CAD build for the part. Positions are in the model's coordinates, mm. Face numbers are marked on the shaded views. A direction names the side the tool comes from. Coordinates: 2 decimals unless noted, no trailing zeros. Answer as CSV lines item,"result". Start each with the question number.
```python
from build123d import *

# Parameters (mm, degrees)
CHAMFER1_SIZE       = 0.5
CHAMFER2_SIZE       = 0.8
SKETCH3_R           = 40.418258265
SKETCH3_R_2         = 4.375
BOSS_EXTRUDE1_DEPTH = 6.7
CHAMFER3_SIZE       = 1.5


with BuildPart() as part:
    # Sketch1 → Revolve1 (revolve)
    with BuildSketch(Plane(origin=(0, 0, 0), x_dir=(1, 0, 0), z_dir=(0, 1, 0)), mode=Mode.PRIVATE) as revolve1_sk:
        Polygon((37.9, 0), (37.9, -8.7), (48, -8.7), (48, -18.7), (51, -18.7), (51, -16.2), (50, -16.2), (50, -11.2), (51, -11.2), (51, -8.7), (52, -8.7), (52, -6.7), (39.9, -6.7), (39.9, 0), align=None)
    revolve(revolve1_sk.sketch.rotate(Axis((0, 0, -73.981367368), (0, 0, 1)), 180), axis=Axis((0, 0, -73.981367368), (0, 0, 1)))

    # Chamfer1
    chamfer1_edges = [part.edges().sort_by_distance(p)[0] for p in [
        (51, 0, 11.2),
        (50, 0, 11.2),
        (50, 0, 16.2),
        (51, 0, 16.2),
        (51, 0, 18.7),
        (39.9, 0, 0),
    ]]
    chamfer(chamfer1_edges, length=CHAMFER1_SIZE - 0.0001)  # a hair under: the kernel refuses the full size

    # Chamfer2
    chamfer2_edges = [part.edges().sort_by_distance(p)[0] for p in [
        (51, 0, 8.7),
    ]]
    chamfer(chamfer2_edges, length=CHAMFER2_SIZE)

    # Sketch3 → Boss-Extrude1 (add)
    with BuildSketch(Plane(origin=(0, 0, 6.7), x_dir=(-1, 0, 0), z_dir=(0, 0, -1))):
        with Locations(Location((0.518258265, 0, 0), (0, 0, 180))):
            Circle(SKETCH3_R)
        with Locations(Location((0.518258265, 0, 0), (0, 0, 180))):
            Circle(SKETCH3_R_2, mode=Mode.SUBTRACT)
    extrude(amount=BOSS_EXTRUDE1_DEPTH)

    # Chamfer3
    chamfer3_edges = [part.edges().sort_by_distance(p)[0] for p in [
        (-4.893258265, 0, 0),
    ]]
    chamfer(chamfer3_edges, length=CHAMFER3_SIZE)


solid = part.part
```
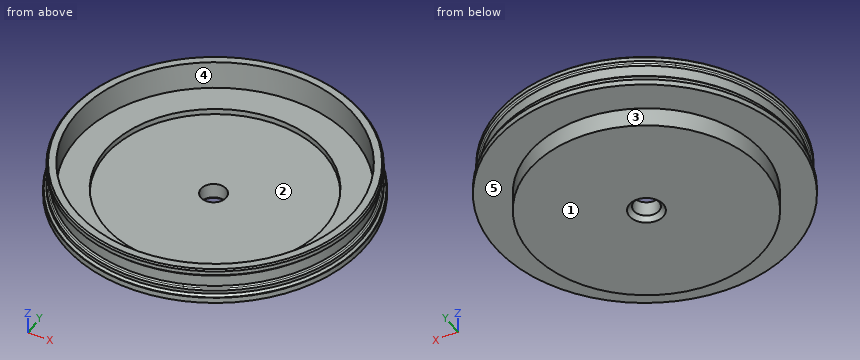
1) Tool access for the marked faces 1 and 2: list every direction of +Z, -Z, +X, -X, +Y, -Y with a clear straight run to the whole face (end or side of a thin tool).
2) Probe L1, parallel to Y at x = 6.5, z = 12.25; L2, parallel to X at y = -24, z = 7.5; L3, parallel to Z at x = -9, y = -10. List the from-to ranges inside material, lowest first. Write a range as [from, to].
3) Pin check, flat tips, straight feed: P1, Ø4, axis at x = -26, z = 9, coming from the -Y side; P2, Ø5, axis at y = 41, z = 8, coming from the +X side; P3, Ø1.5, axis at x = -29.5, y = -40.5, coming from the -Z side; P4, Ø14, axis at x = -0.52, y = 0, coming from the -Z side. Stop position of each tip, or through.
4) Two-plate mould, pull along X, no slides. Class the marked faces 3, 4 and 5: pulls with the +X half, pulls with the -X half, needs draft (parallel to the pull), parting line crosses it, or undercut.
Result sheet:
1,face 1,"-Z, +X, -X, +Y, -Y"
1,face 2,"+Z"
2,L1,"y = [-49.58, -47.56], [47.56, 49.58]"
2,L2,"x = [-46.13, -29.33], [29.33, 46.13]"
2,L3,"z = [0, 6.7]"
3,P1,"stops at y = -46.12"
3,P2,"stops at x = 34.95"
3,P3,"stops at z = 6.7"
3,P4,"stops at z = 0"
4,face 3,"parting line crosses it"
4,face 4,"undercut"
4,face 5,"needs draft"
